The listing builds one solid part. Answer for the finished solid, in the listing's coordinates (mm). A direction names the side the tool comes from. Round coordinates to 2 decimals unless told otherwise and drop trailing zeros. Write each loop counter-clockwise with the first axis right and the second up, starting at its lowest first coordinate (ties: lowest second). Pieces come first, ordered by that corner, then holes. Notation, with made-up numbers: (3.25, -37.75) -> (26.25, -37.75) arc R9 cw to (26.25, -25.75) -> close; hole circle Ø1 at (66, 88). An arc over 180 degrees is marked (long way). Write each question's results on one line, items separated by ' | '. Start each with the question number.
```python
from build123d import *

# Parameters (mm, degrees)
SALIENTE_EXTRUIR1_DEPTH    = 35
CROQUIS3_R                 = 1.5
CORTAR_EXTRUIR2_DEPTH      = 38.749172176
CROQUIS6_W                 = 15
CROQUIS6_H                 = 20
CORTAR_EXTRUIR4_DEPTH      = 20
CORTAR_EXTRUIR5_DEPTH      = 38.749172176
CORTAR_EXTRUIR5_DEPTH_BACK = 38.749172176
CROQUIS7_R                 = 1.5
CORTAR_EXTRUIR1_DEPTH      = 38.749172328
CORTAR_EXTRUIR1_DEPTH_BACK = 38.749172328
CORTAR_EXTRUIR3_DEPTH      = 38.749172461
CORTAR_EXTRUIR3_DEPTH_BACK = 38.749172461
CUT_EXTRUDE1_DEPTH         = 4
SKETCH2_R                  = 3
BOSS_EXTRUDE1_DEPTH        = 2
SKETCH3_R                  = 4
BOSS_EXTRUDE2_DEPTH        = 2
FILLET1_R                  = 1
FILLET2_R                  = 1
FILLET4_R                  = 1


with BuildPart() as part:
    # Croquis1 → Saliente-Extruir1 (new body)
    with BuildSketch(Plane.XY):
        with BuildLine():
            Line((-7.5, 10), (7.5, 10))
            ThreePointArc((7.5, 10), (10, 0), (7.5, -10))
            Line((7.5, -10), (-7.5, -10))
            ThreePointArc((-7.5, -10), (-10, 0), (-7.5, 10))
        make_face()
    extrude(amount=SALIENTE_EXTRUIR1_DEPTH)

    # Croquis3 → Cortar-Extruir2 (cut, through all)
    with BuildSketch(Plane.XY.offset(35)):
        with Locations((0, -7)):
            Circle(CROQUIS3_R)
    extrude(amount=-CORTAR_EXTRUIR2_DEPTH, mode=Mode.SUBTRACT)

    # Croquis6 → Cortar-Extruir4 (cut)
    with BuildSketch(Plane.XY.offset(35)):
        Rectangle(CROQUIS6_W, CROQUIS6_H)
    extrude(amount=-CORTAR_EXTRUIR4_DEPTH, mode=Mode.SUBTRACT)

    # Croquis7 → Cortar-Extruir5 (cut, two sides: drawn at the far end of the back side and taken through both)
    with BuildSketch(Plane(origin=(0, 0, 0), x_dir=(0, 0, -1), z_dir=(1, 0, 0)).offset(-CORTAR_EXTRUIR5_DEPTH_BACK)):
        with Locations((-25, 0)):
            Circle(CROQUIS7_R)
        with BuildLine():
            Line((-25, -10), (-41, -10))
            Line((-41, -10), (-41, 10))
            Line((-41, 10), (-25, 10))
            ThreePointArc((-25, 10), (-35, 0), (-25, -10))
        make_face()
    extrude(amount=CORTAR_EXTRUIR5_DEPTH + CORTAR_EXTRUIR5_DEPTH_BACK, mode=Mode.SUBTRACT)

    # Croquis2 → Cortar-Extruir1 (cut, two sides: drawn at the far end of the back side and taken through both)
    with BuildSketch(Plane(origin=(0, 0, 0), x_dir=(1, 0, 0), z_dir=(0, 1, 0)).offset(-CORTAR_EXTRUIR1_DEPTH_BACK)):
        with BuildLine():
            Line((-1.261783996, 0), (1.261783996, 0))
            add(Edge.make_bspline(
                [(10, -17.5), (10, -1.960721315), (1.261783996, 0)],
                knots=[4.71238898, 4.71238898, 4.71238898, 6.156669672, 6.156669672, 6.156669672], degree=2, weights=[1, 0.750392697, 1]))
            Line((10, -17.5), (10, 3.270111557))
            Line((10, 3.270111557), (-10, 3.270111557))
            Line((-10, 3.270111557), (-10, -17.5))
            add(Edge.make_bspline(
                [(-1.261783996, 0), (-10, -1.960721315), (-10, -17.5)],
                knots=[0.126515635, 0.126515635, 0.126515635, 1.570796327, 1.570796327, 1.570796327], degree=2, weights=[1, 0.750392697, 1]))
        make_face()
    extrude(amount=CORTAR_EXTRUIR1_DEPTH + CORTAR_EXTRUIR1_DEPTH_BACK, mode=Mode.SUBTRACT)

    # Croquis5 → Cortar-Extruir3 (cut, two sides: drawn at the far end of the back side and taken through both)
    with BuildSketch(Plane(origin=(0, 0, 0), x_dir=(0, 0, -1), z_dir=(1, 0, 0)).offset(-CORTAR_EXTRUIR3_DEPTH_BACK)):
        with BuildLine():
            Line((-17.5, -10), (6.249957369, -10))
            Line((6.249957369, -10), (6.249957369, 10))
            Line((6.249957369, 10), (-17.5, 10))
            add(Edge.make_bspline(
                [(-17.5, -10), (0, -10), (0, 0), (0, 10), (-17.5, 10)],
                knots=[4.71238898, 4.71238898, 4.71238898, 6.283185307, 6.283185307, 7.853981634, 7.853981634, 7.853981634], degree=2, weights=[1, 0.707106781, 1, 0.707106781, 1]))
        make_face()
    extrude(amount=CORTAR_EXTRUIR3_DEPTH + CORTAR_EXTRUIR3_DEPTH_BACK, mode=Mode.SUBTRACT)

    # Sketch1 → Cut-Extrude1 (cut)
    with BuildSketch(Plane(origin=(0, 10, 0), x_dir=(1, 0, 0), z_dir=(0, 1, 0))):
        with BuildLine():
            Line((-6, -9), (-6, -15))
            Line((-6, -15), (6, -15))
            Line((6, -15), (6, -9))
            ThreePointArc((6, -9), (0, -3), (-6, -9))
        make_face()
    extrude(amount=-CUT_EXTRUDE1_DEPTH, mode=Mode.SUBTRACT)

    # Sketch2 → Boss-Extrude1 (add)
    with BuildSketch(Plane(origin=(0, 6, 0), x_dir=(1, 0, 0), z_dir=(0, 1, 0))):
        with Locations(Location((0, -9, 0), (0, 0, 270))):
            Circle(SKETCH2_R)
    extrude(amount=BOSS_EXTRUDE1_DEPTH)

    # Sketch3 → Boss-Extrude2 (add)
    with BuildSketch(Plane(origin=(0, 8, 0), x_dir=(1, 0, 0), z_dir=(0, 1, 0))):
        with Locations(Location((0, -9, 0), (0, 0, 270))):
            Circle(SKETCH3_R)
    extrude(amount=BOSS_EXTRUDE2_DEPTH)

    # Fillet1
    fillet1_edges = [part.edges().sort_by_distance(p)[0] for p in [
        (0, 6, 6),
        (0, 8, 6),
    ]]
    fillet(fillet1_edges, radius=FILLET1_R - 0.0001)  # a hair under: the kernel refuses the full size

    # Fillet2
    fillet2_edges = [part.edges().sort_by_distance(p)[0] for p in [
        (0, 6, 15),
    ]]
    fillet(fillet2_edges, radius=FILLET2_R)

    # Fillet4
    fillet4_edges = [part.edges().sort_by_distance(p)[0] for p in [
        (-1.5, -7, 15),
    ]]
    fillet(fillet4_edges, radius=FILLET4_R)


solid = part.part
```
Q1. The part is cut by section A-A, the plane z = 31. Write down the section's boundary in (x, y), then the cut area to 3 significant figures.
Q2. Each of these flat-tipped pins is pushed along its axis until it touches: pin 1 (4 mm diameter, centred on x = -7, y = -7.5, fed in from -Z); pin 2 (3 mm diameter, centred on y = 3.5, z = 12.5, fed in from -X); pin 3 (6.5 mm diameter, centred on x = 1.5, z = 7.5, fed in from -Y). Where does it stop, or does it pass through?
Q3. Determine the mould class of faces 6 (the cylindrical face through (-8, 0, 35)), 7 (the flat face through (-6, 8, 12)), 8 (the cylindrical face through (-8.77, 0.07, 26.5)) for opening direction Z: pulls with the +Z half, pulls with the -Z half, needs draft (parallel to the pull), parting line crosses it, or undercut.
Q4. The part is cut by section B-B, the plane y = 0. State how many separate pieces and enclosed holes the cut face has, then the cut area to 3 significant figures.
Q5. For faces 1 (the flat face through (6, 8, 12)), 2 (the flat face through (3, 6, 12)), 3 (the cylindrical face through (8.73, 0.07, 26.5)), 4 (the flat face through (7.5, 0, 23)), 5 (the cylindrical face through (-10, 0, 21)), determine the directions among +Z, -Z, +X, -X, +Y, -Y from which every point of the face is accessible in a straight line to the end or side of a thin tool.
Q6. Find the intervals of material crossed by line 1 (Z direction, x = -6.25, y = -7); line 2 (X direction, y = 3.75, z = 16); line 3 (X direction, y = -0.75, z = 30.5), in increasing order.
Answers follow:
1) outline: (-8.44, -8) -> (-7.5, -8) -> (-7.5, 8) -> (-8.44, 8) arc R21.25 ccw to start; (7.5, -8) -> (8.44, -8) arc R21.25 ccw to (8.44, 8) -> (7.5, 8) -> close | area: 63.6 mm^2
2) pin 1: z = 3.27 | pin 2: x = -9.79 | pin 3: y = -9.23
3) face 6: pulls with the +Z half | face 7: needs draft | face 8: undercut
4) separate pieces: 3 | enclosed holes: 0 | area: 312 mm^2
5) face 1: +Z, +Y | face 2: +Y | face 3: +X, -X | face 4: +Z, +Y, -Y | face 5: +Z, -Z, -X
6) line 1: 5 to 15 | line 2: -9.67 to -7.5, 7.5 to 9.67 | line 3: -9.99 to -7.5, 7.5 to 9.99
